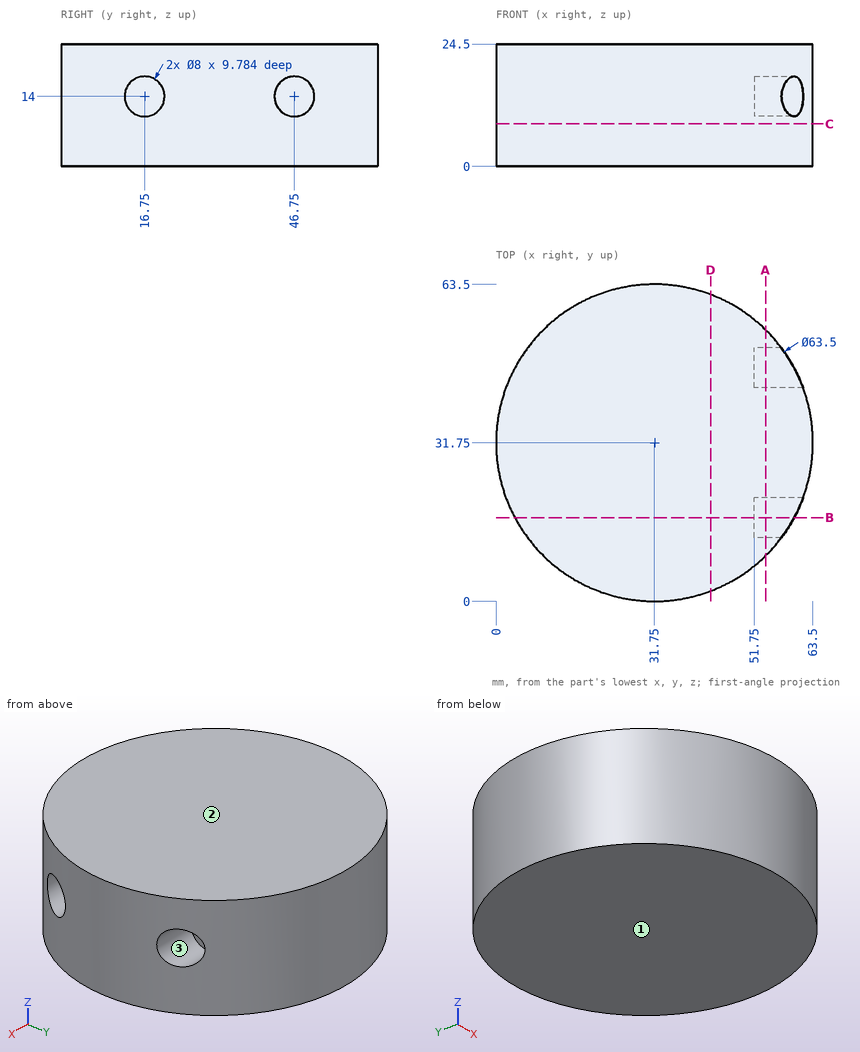
Design review of the part shown in the three views and the two pictorial views. Dimensions are in mm from the part's minimum x, y and z. Round coordinates to 2 decimals unless told otherwise and drop trailing zeros. Write each loop counter-clockwise with the first axis right and the second up, starting at its lowest first coordinate (ties: lowest second). Pieces come first, ordered by that corner, then holes.
Item 1: Clearance check with flat-ended pins moving along their axes: pin 1 Ø1 at (y, z) = (10, 18.5) entering from +X; pin 2 Ø4 at (x, z) = (53.5, 22) entering from -Y; pin 3 Ø3 at (x, z) = (24.5, 16.5) entering from -Y (1 decimal). State where each tip first meets the part, or that it passes through.
Item 2: We need section C-C on z = 8.5. Write out the cut boundary in (x, y).
Item 3: The part is to be moulded in two halves that separate along Z. For the marked faces 1, 2 and 3, say which applies: +Z half, -Z half, draft (parallel to the pull), parting line (faces both ways), or undercut.
Item 4: For probe 1 along Y at (x, z) = (55, 14); probe 2 along Y at (x, z) = (58, 14); probe 3 along Z at (x, y) = (59, 46), list the stretches that pass through material, from the lowest coordinate up.
Item 5: We need section B-B on y = 16.75. Write out the cut boundary in (x, z).
Item 6: We need section D-D on x = 43. Write out the cut boundary in (y, z), and give its area (3 significant figures).
Item 7: We need section A-A on x = 54. Write out the cut boundary in (y, z), and give its area (3 significant figures).
Returned:
1. pin 1: stops at x = 55.34
1. pin 2: stops at y = 6.89
1. pin 3: stops at y = 0.5
2. outline: circle Ø63.5 at (31.75, 31.75)
3. face 1: -Z half
3. face 2: +Z half
3. face 3: undercut
4. probe 1: y = 10.13 to 12.75, 20.75 to 42.75, 50.75 to 53.37
4. probe 2: y = 20.75 to 42.75
4. probe 3: z = 0 to 10.07, 17.93 to 24.5
5. outline: (3.77, 0) - (59.73, 0) - (59.73, 10) - (51.75, 10) - (51.75, 18) - (59.73, 18) - (59.73, 24.5) - (3.77, 24.5) - close
6. outline: (2.06, 0) - (61.44, 0) - (61.44, 24.5) - (2.06, 24.5) - close
6. area: 1,450 mm2
7. outline: (9.1, 0) - (54.4, 0) - (54.4, 24.5) - (9.1, 24.5) - close; hole circle Ø8 at (16.75, 14); hole circle Ø8 at (46.75, 14)
7. area: 1,010 mm2
